For this review, take the finished solid that the model builds, in its own axes (mm). Face numbers are marked on the shaded views. A direction names the side the tool comes from. Round coordinates to 2 decimals unless told otherwise and drop trailing zeros. Write each loop counter-clockwise with the first axis right and the second up, starting at its lowest first coordinate (ties: lowest second). Pieces come first, ordered by that corner, then holes.
from build123d import *

# Parameters (mm, degrees)
BOSS_EXTRUDE1_DEPTH    = 50.8
CONVERT_SOLID3_DEPTH   = 50.8
CONVERT_SOLID3_2_DEPTH = 50.8


# Read off the part's stored shape, not the designer's step: Convert-Solid3
with BuildPart() as part:
    # Sketch1 → Boss-Extrude1 (new body)
    with BuildSketch(Plane(origin=(0, 0, 0), x_dir=(1, 0, 0), z_dir=(0, 1, 0))):
        Polygon((-9.94664, 28.15336), (15.45336, 28.15336), (15.45336, -22.64664), (38.1, -22.64664), (38.1, -25.4), (12.7, -25.4), (12.7, 25.4), (-12.7, 25.4), (-12.7, 50.8), (-9.94664, 50.8), align=None)
    extrude(amount=BOSS_EXTRUDE1_DEPTH)

    # Convert-Solid3 outline → Convert-Solid3 (cut)
    with BuildSketch(Plane(origin=(0, 0, 0), x_dir=(1, 0, 0), z_dir=(0, 1, 0))):
        with BuildLine():
            ThreePointArc((11.7, 28.15336), (14.354026308, 27.054026308), (15.45336, 24.4))
            Line((15.45336, 24.4), (15.45336, 28.15336))
            Line((15.45336, 28.15336), (11.7, 28.15336))
        make_face()
        with BuildLine():
            Line((-12.7, 25.4), (-8.94664, 25.4))
            ThreePointArc((-8.94664, 25.4), (-11.600666308, 26.499333692), (-12.7, 29.15336))
            Line((-12.7, 29.15336), (-12.7, 25.4))
        make_face()
        with BuildLine():
            ThreePointArc((16.45336, -25.4), (13.799333692, -24.300666308), (12.7, -21.64664))
            Line((12.7, -21.64664), (12.7, -25.4))
            Line((12.7, -25.4), (16.45336, -25.4))
        make_face()
    extrude(amount=CONVERT_SOLID3_DEPTH, mode=Mode.SUBTRACT)

    # Convert-Solid3 2 outline → Convert-Solid3 2 (add)
    with BuildSketch(Plane(origin=(0, 0, 0), x_dir=(1, 0, 0), z_dir=(0, 1, 0))):
        with BuildLine():
            Line((-9.94664, 28.15336), (-8.94664, 28.15336))
            ThreePointArc((-8.94664, 28.15336), (-9.653746781, 28.446253219), (-9.94664, 29.15336))
            Line((-9.94664, 29.15336), (-9.94664, 28.15336))
        make_face()
        with BuildLine():
            ThreePointArc((16.45336, -22.64664), (15.746253219, -22.353746781), (15.45336, -21.64664))
            Line((15.45336, -21.64664), (15.45336, -22.64664))
            Line((15.45336, -22.64664), (16.45336, -22.64664))
        make_face()
        with BuildLine():
            ThreePointArc((11.7, 25.4), (12.407106781, 25.107106781), (12.7, 24.4))
            Line((12.7, 24.4), (12.7, 25.4))
            Line((12.7, 25.4), (11.7, 25.4))
        make_face()
    extrude(amount=CONVERT_SOLID3_2_DEPTH)


solid = part.part
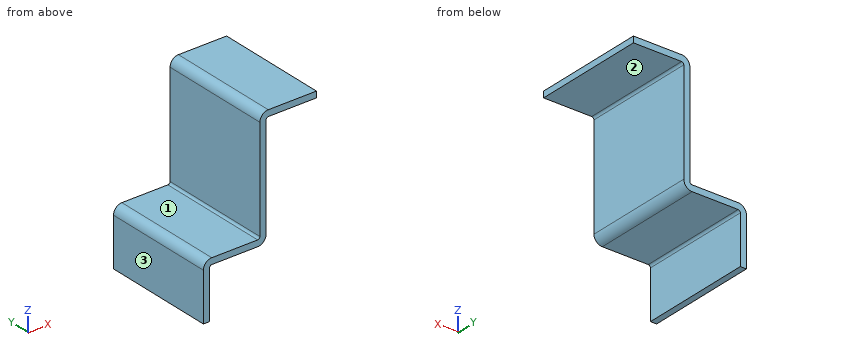
(1) For line 1 along Z through (x, y) = (3, 38.5); line 2 along Z through (x, y) = (22, 2.5); line 3 along X through (y, z) = (12.5, 5.5), list the stretches that pass through material, from the lowest coordinate up.
Geometry check:
line 1: z = -28.15 to -25.4
line 2: z = 22.65 to 25.4
line 3: x = 12.7 to 15.45
(2) For the marked faces 1, 2 and 3, list the 3-axis set-ups (+Z, -Z, +X, -X, +Y, -Y) from which the entire face can be reached by the end or side of a thin tool; tool diameter is ignored.
Geometry check:
face 1: +Z, -X, +Y, -Y
face 2: -Z, +X, +Y, -Y
face 3: +Z, -Z, -X, +Y, -Y
(3) We need section A-A, the plane y = 24.5. Give the boundary of the cut face in (x, z), and give its area (3 significant figures).
Geometry check:
outline: (-12.7, -50.8) - (-9.95, -50.8) - (-9.95, -29.15) arc R1 cw to (-8.95, -28.15) - (11.7, -28.15) arc R3.75 ccw to (15.45, -24.4) - (15.45, 21.65) arc R1 cw to (16.45, 22.65) - (38.1, 22.65) - (38.1, 25.4) - (16.45, 25.4) arc R3.75 ccw to (12.7, 21.65) - (12.7, -24.4) arc R1 cw to (11.7, -25.4) - (-8.95, -25.4) arc R3.75 ccw to (-12.7, -29.15) - close
area: 334 mm2
(4) We need section B-B, the plane z = 0. Give the boundary of the cut face in (x, y).
Geometry check:
outline: (12.7, 0) - (15.45, 0) - (15.45, 50.8) - (12.7, 50.8) - close
(5) For pin 1 Ø22.5 at (x, y) = (-2.5, 34) entering from +Z; pin 2 Ø24 at (x, y) = (24.5, 24.5) entering from -Z; pin 3 Ø3 at (y, z) = (45, -6) entering from +X, all flat-tipped, find the tip position at first contact; note any pin that passes through.
Geometry check:
pin 1: stops at z = -25.4
pin 2: stops at z = -28.07
pin 3: stops at x = 15.45
(6) We need section C-C, the plane x = -4.5. Give the boundary of the cut face in (y, z), and give its area (3 significant figures).
Geometry check:
outline: (0, -28.15) - (50.8, -28.15) - (50.8, -25.4) - (0, -25.4) - close
area: 140 mm2
